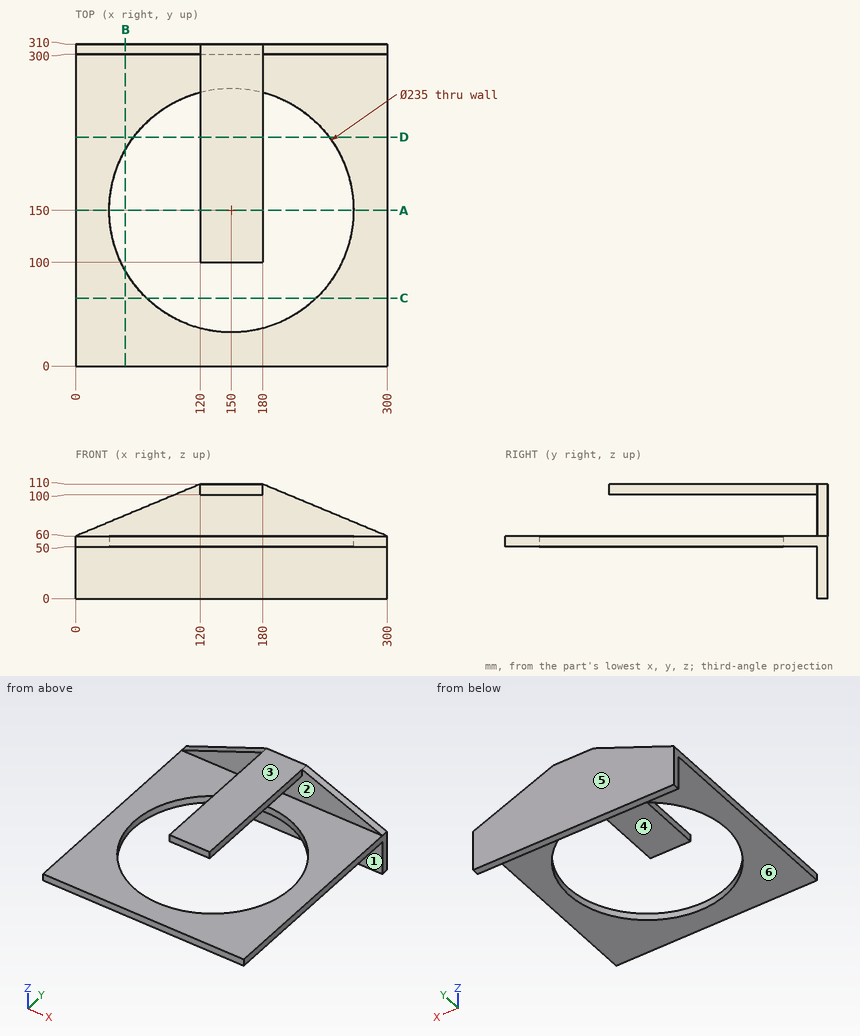
Print and shaded views of the part. All mm, measured from the part's lowest x, y and z. A direction names the side the tool comes from. Coordinates: 2 decimals unless noted, no trailing zeros. Write each loop counter-clockwise with the first axis right and the second up, starting at its lowest first coordinate (ties: lowest second). Pieces come first, ordered by that corner, then holes.
(1) Drill centre lines: probe 1 along X at (y, z) = (150, 53); probe 2 along Y at (x, z) = (150, 56.5); probe 3 along Y at (x, z) = (121, 35). Where is each one in solid material? Low to high.
(2) Cut at A-A, the plane y = 150. List the corners of the cut face in (x, z), and give its area (3 significant figures).
(3) Cut at B-B, the plane x = 48. List the corners of the cut face in (y, z).
(4) Cut at D-D, the plane y = 220.5. List the corners of the cut face in (x, z), and give its area (3 significant figures).
(5) 3-axis set-ups, long thin cutter, end or side, ignore diameter. For the marked faces 4, 5 and 6: which of +Z, -Z, +X, -X, +Y, -Y reach the whole face in a straight line?
(6) Flat gauge pins, fed straight in: pin 1 (11 mm diameter, centred on y = 208, z = 107.5, fed in from -X); pin 2 (5 mm diameter, centred on x = 157, z = 103.5, fed in from -Y); pin 3 (1 mm diameter, centred on x = 183.5, z = 20.5, fed in from -Y); pin 4 (10 mm diameter, centred on x = 268.5, z = 63.5, fed in from -Y). Where does each tip first touch, or does it go through?
(7) Cut at C-C, the plane y = 65.5. List the corners of the cut face in (x, z).
(8) Two-plate mould, pull along Z, no slides. Class the marked faces 1, 2 and 3: +Z half, -Z half, draft (parallel to the pull), parting line (faces both ways), or undercut.
Geometry says:
1. probe 1: x = 0 to 32.5, 267.5 to 300
1. probe 2: y = 0 to 32.5, 267.5 to 310
1. probe 3: y = 300 to 310
2. outline: (0, 50) - (32.5, 50) - (32.5, 60) - (0, 60) - close; (120, 100) - (180, 100) - (180, 110) - (120, 110) - close; (267.5, 50) - (300, 50) - (300, 60) - (267.5, 60) - close
2. area: 1,250 mm2
3. outline: (0, 50) - (91.67, 50) - (91.67, 60) - (0, 60) - close; (208.33, 50) - (300, 50) - (300, 0) - (310, 0) - (310, 80) - (300, 80) - (300, 60) - (208.33, 60) - close
4. outline: (0, 50) - (56, 50) - (56, 60) - (0, 60) - close; (120, 100) - (180, 100) - (180, 110) - (120, 110) - close; (244, 50) - (300, 50) - (300, 60) - (244, 60) - close
4. area: 1,720 mm2
5. face 4: +X, -X, -Y
5. face 5: +Z, -Z, +X, -X, +Y
5. face 6: -Z, +X, -X, -Y
6. pin 1: stops at x = 120
6. pin 2: stops at y = 100
6. pin 3: stops at y = 300
6. pin 4: stops at y = 0
7. outline: (0, 50) - (68.35, 50) - (68.35, 60) - (0, 60) - close; (231.65, 50) - (300, 50) - (300, 60) - (231.65, 60) - close
8. face 1: draft
8. face 2: undercut
8. face 3: +Z half
